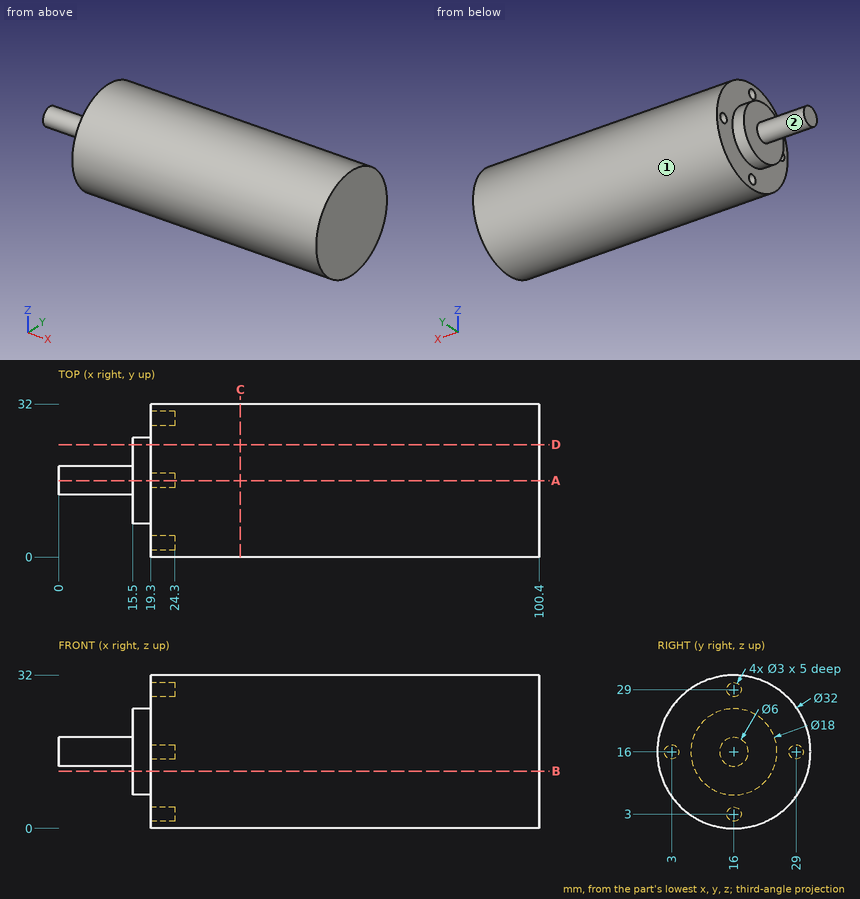
Part print with two shaded views. Sizes in mm from the minimum x, y, z corner. A direction names the side the tool comes from. Round coordinates to 2 decimals unless told otherwise and drop trailing zeros. Order: outer loops, then holes, each group sorted by start corner. A loop starts at its lowest first (then second) coordinate and runs counter-clockwise, first axis right, second up.
(1) Band-saw the part on B-B (z = 12). List the corners of the cut face in (x, y), then the cut area to 3 significant figures.
(2) Band-saw the part on D-D (y = 23.5). List the corners of the cut face in (x, z), then the cut area to 3 significant figures.
(3) 3-axis set-ups, long thin cutter, end or side, ignore diameter. For the marked faces 1 and 2: which of +Z, -Z, +X, -X, +Y, -Y reach the whole face in a straight line?
(4) Band-saw the part on A-A (y = 16). List the corners of the cut face in (x, z), then the cut area to 3 significant figures.
(5) Pin check, flat tips, straight feed: pin 1 (4 mm diameter, centred on x = 30, z = 8.5, fed in from +Y) (3 decimals); pin 2 (3 mm diameter, centred on x = 41, z = 7, fed in from -Y); pin 3 (4 mm diameter, centred on x = 51.5, y = 6.5, fed in from +Z). Stop position of each tip, or through.
(6) Band-saw the part on C-C (x = 38). List the corners of the cut face in (y, z), then the cut area to 3 significant figures.
(7) Drill centre lines: line 1 (X direction, y = 3, z = 7.5); line 2 (X direction, y = 20, z = 18); line 3 (Y direction, x = 21.2, z = 3). Where is each one in solid material? Low to high.
Verdict:
1. outline: (15.5, 7.94) - (19.3, 7.94) - (19.3, 0.51) - (100.4, 0.51) - (100.4, 31.49) - (19.3, 31.49) - (19.3, 24.06) - (15.5, 24.06) - close
1. area: 2,570 mm2
2. outline: (15.5, 11.03) - (19.3, 11.03) - (19.3, 1.87) - (100.4, 1.87) - (100.4, 30.13) - (19.3, 30.13) - (19.3, 20.97) - (15.5, 20.97) - close
2. area: 2,330 mm2
3. face 1: +X, -X
3. face 2: -X
4. outline: (0, 13) - (15.5, 13) - (15.5, 7) - (19.3, 7) - (19.3, 4.5) - (24.3, 4.5) - (24.3, 1.5) - (19.3, 1.5) - (19.3, 0) - (100.4, 0) - (100.4, 32) - (19.3, 32) - (19.3, 30.5) - (24.3, 30.5) - (24.3, 27.5) - (19.3, 27.5) - (19.3, 25) - (15.5, 25) - (15.5, 19) - (0, 19) - close
4. area: 2,730 mm2
5. pin 1: stops at y = 31.025
5. pin 2: stops at y = 1.87
5. pin 3: stops at z = 30.13
6. outline: circle Ø32 at (16, 16)
6. area: 804 mm2
7. line 1: x = 19.3 to 100.4
7. line 2: x = 15.5 to 100.4
7. line 3: y = 6.67 to 14.5, 17.5 to 25.33
